CAD build for the part. Positions are in the model's coordinates, mm. Face numbers are marked on the shaded views. A direction names the side the tool comes from. Give positions to 0.01 mm unless a question says otherwise; leave off trailing zeros. Write each loop counter-clockwise with the first axis right and the second up, starting at its lowest first coordinate (ties: lowest second). Pieces come first, ordered by that corner, then holes. Notation, with made-up numbers: (-10.75, 67) -> (6.25, 67) arc R27 cw to (6.25, 89) -> close; hole circle Ø11 at (-24, 11.25). An arc over 180 degrees is marked (long way). Use one line per item in the form item = value. Start each with the question number.
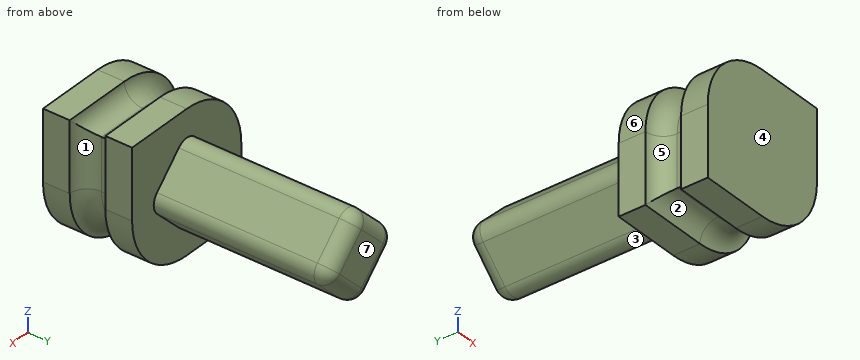
from build123d import *

# Parameters (mm, degrees)
BOSS_EXTRUDE1_DEPTH     = 5
BOSS_EXTRUDE2_DEPTH     = 9.8
CUT_EXTRUDE2_DEPTH      = 1
CUT_EXTRUDE2_DEPTH_BACK = 1
FILLET1_R               = 1
FILLET3_R               = 0.8


with BuildPart() as part:
    # Sketch1 → Boss-Extrude1 (new body)
    with BuildSketch(Plane(origin=(0, 0, 0), x_dir=(1, 0, 0), z_dir=(0, 1, 0))):
        with BuildLine():
            Line((-3.9, 3.9), (0, 3.9))
            ThreePointArc((0, 3.9), (2.757716447, 2.757716447), (3.9, 0))
            Line((3.9, 0), (3.9, -3.9))
            Line((3.9, -3.9), (0, -3.9))
            ThreePointArc((0, -3.9), (-2.757716447, -2.757716447), (-3.9, 0))
            Line((-3.9, 0), (-3.9, 3.9))
        make_face()
    extrude(amount=BOSS_EXTRUDE1_DEPTH)

    # Sketch2 → Boss-Extrude2 (add)
    with BuildSketch(Plane(origin=(0, 5, 0), x_dir=(1, 0, 0), z_dir=(0, 1, 0))):
        with BuildLine():
            Line((-0.565685425, 2.121320344), (-2.121320344, 0.565685425))
            ThreePointArc((-2.121320344, 0.565685425), (-2.355634919, 0), (-2.121320344, -0.565685425))
            Line((-2.121320344, -0.565685425), (-0.565685425, -2.121320344))
            ThreePointArc((-0.565685425, -2.121320344), (0, -2.355634919), (0.565685425, -2.121320344))
            Line((0.565685425, -2.121320344), (2.121320344, -0.565685425))
            ThreePointArc((2.121320344, -0.565685425), (2.355634919, 0), (2.121320344, 0.565685425))
            Line((2.121320344, 0.565685425), (0.565685425, 2.121320344))
            ThreePointArc((0.565685425, 2.121320344), (0, 2.355634919), (-0.565685425, 2.121320344))
        make_face()
    extrude(amount=BOSS_EXTRUDE2_DEPTH)

    # Sketch3 → Cut-Extrude2 (cut, two sides: drawn at the far end of the back side and taken through both)
    with BuildSketch(Plane(origin=(0, 2.5, 0), x_dir=(1, 0, 0), z_dir=(0, 1, 0)).offset(-CUT_EXTRUDE2_DEPTH_BACK)):
        with BuildLine():
            Line((-3.9, 0), (-3.9, 3.9))
            Line((-3.9, 3.9), (0, 3.9))
            ThreePointArc((0, 3.9), (2.757716447, 2.757716447), (3.9, 0))
            Line((3.9, 0), (3.9, -3.9))
            Line((3.9, -3.9), (0, -3.9))
            ThreePointArc((0, -3.9), (-2.757716447, -2.757716447), (-3.9, 0))
        make_face()
        with BuildLine():
            Line((-2.9, 0), (-2.9, 2.9))
            Line((-2.9, 2.9), (0, 2.9))
            ThreePointArc((0, 2.9), (2.050609665, 2.050609665), (2.9, 0))
            Line((2.9, 0), (2.9, -2.9))
            Line((2.9, -2.9), (0, -2.9))
            ThreePointArc((0, -2.9), (-2.050609665, -2.050609665), (-2.9, 0))
        make_face(mode=Mode.SUBTRACT)
    extrude(amount=CUT_EXTRUDE2_DEPTH + CUT_EXTRUDE2_DEPTH_BACK, mode=Mode.SUBTRACT)

    # Fillet1
    fillet1_edges = [part.edges().sort_by_distance(p)[0] for p in [
        (2.9, 3.5, 1.45),
        (2.050609665, 3.5, -2.050609665),
        (1.45, 3.5, 2.9),
        (-2.050609665, 3.5, 2.050609665),
        (2.9, 1.5, 1.45),
        (2.050609665, 1.5, -2.050609665),
        (-2.9, 1.5, -1.45),
        (1.45, 1.5, 2.9),
        (-1.45, 3.5, -2.9),
        (-2.9, 3.5, -1.45),
        (-1.45, 1.5, -2.9),
        (-2.050609665, 1.5, 2.050609665),
    ]]
    fillet(fillet1_edges, radius=FILLET1_R - 0.0001)  # a hair under: the kernel refuses the full size

    # Fillet3
    fillet3_edges = [part.edges().sort_by_distance(p)[0] for p in [
        (0, 14.8, 2.355634919),
        (1.343502884, 14.8, 1.343502884),
        (2.355634919, 14.8, 0),
        (1.343502884, 14.8, -1.343502884),
        (0, 14.8, -2.355634919),
        (-1.343502884, 14.8, -1.343502884),
        (-2.355634919, 14.8, 0),
        (-1.343502884, 14.8, 1.343502884),
    ]]
    fillet(fillet3_edges, radius=FILLET3_R)


solid = part.part
1) Pin check, flat tip, straight feed: pin 1 (1.5 mm diameter, centred on x = 1.5, y = 7, fed in from +Z). Stop position of the tip, or through.
2) Cut at A-A (y = 11). Give the cut face in (x, z), and give its area (3 significant figures).
3) 3-axis set-ups, long thin cutter, end or side, ignore diameter. For the marked faces 1, 2 and 3: which of +Z, -Z, +X, -X, +Y, -Y reach the whole face in a straight line?
4) Cut at B-B (y = 2.75). Give the cut face in (x, z), and give its area (3 significant figures).
5) Wall check: line 1 along Y through (x, z) = (1.75, -2); line 2 along Y through (x, z) = (2, -2.5); line 3 along Y through (x, z) = (2, 3.75). Give the ranges that are in metal, low to high. Write a range as from..to.
6) Two-plate mould, pull along Y, no slides. Class the marked faces 4, 5, 6 and 7: released by +Y, released by -Y, zero draft, split by the parting line, or undercut.
Final values:
q1.pin_1 = 1.94
q2.outline = (-2.12, -0.57) -> (-0.57, -2.12) arc R0.8 ccw to (0.57, -2.12) -> (2.12, -0.57) arc R0.8 ccw to (2.12, 0.57) -> (0.57, 2.12) arc R0.8 ccw to (-0.57, 2.12) -> (-2.12, 0.57) arc R0.8 ccw to start
q2.area = 13.9 mm^2
q3.face_1 = +Z, -Z, +X
q3.face_2 = -Z, +X, -X
q3.face_3 = -Z, +Y
q4.outline = (-2.93, -2.93) -> (0, -2.93) arc R2.93 ccw to (2.93, 0) -> (2.93, 2.93) -> (0, 2.93) arc R2.93 ccw to (-2.93, 0) -> close
q4.area = 30.7 mm^2
q5.line_1 = 0..5
q5.line_2 = 0..1.78, 3.22..5
q5.line_3 = 0..1.51, 3.49..5
q6.face_4 = released by -Y
q6.face_5 = undercut
q6.face_6 = zero draft
q6.face_7 = released by +Y
